Could you check a few things on this model? Use its own coordinates, in mm. Give positions to 0.01 mm unless a question says otherwise; leave off trailing zeros. Order: outer loops, then holes, each group sorted by start corner. A loop starts at its lowest first (then second) coordinate and runs counter-clockwise, first axis right, second up. Notation, with made-up numbers: (9.5, 41) -> (44.5, 41) arc R11 ccw to (44.5, 52) -> close; hole circle Ø1 at (-3, 64.25). An arc over 180 degrees is marked (long way). Use one line per item in the form item = value. Start each with the question number.
from build123d import *

# Parameters (mm, degrees)
SKETCH1_R                  = 19.05
BOSS_EXTRUDE1_DEPTH        = 7.62
SKETCH2_R                  = 2.54
CUT_EXTRUDE1_DEPTH         = 8.62
F_10_24_TAPPED_HOLE1_D     = 3.7973
CIRPATTERN1_COUNT          = 4
F_10_24_TAPPED_HOLE4_D     = 3.7973
F_10_24_TAPPED_HOLE4_DEPTH = 20.0279
F_10_24_TAPPED_HOLE4_TIP   = 1.140824014


with BuildPart() as part:
    # Sketch1 → Boss-Extrude1 (new body)
    with BuildSketch(Plane.XY):
        Circle(SKETCH1_R)
    extrude(amount=BOSS_EXTRUDE1_DEPTH)

    # Sketch2 → Cut-Extrude1 (cut, through all)
    with BuildSketch(Plane.XY.offset(7.62)):
        Circle(SKETCH2_R)
    extrude(amount=-CUT_EXTRUDE1_DEPTH, mode=Mode.SUBTRACT)

    # #10-24 Tapped Hole1 (through all)
    with Locations(Plane.XY.offset(7.62)):
        with Locations((0, 12.7)):
            f_10_24_tapped_hole1 = Hole(F_10_24_TAPPED_HOLE1_D / 2)

    # CirPattern1: #10-24 Tapped Hole1 ×4 about axis
    cirpattern1_axis = Axis((0, 0, 0), (0, 0, 1))
    for i in range(1, CIRPATTERN1_COUNT):
        add(f_10_24_tapped_hole1.rotate(cirpattern1_axis, i * 360 / CIRPATTERN1_COUNT), mode=Mode.SUBTRACT)

    # #10-24 Tapped Hole4
    with Locations(Plane(origin=(13.470384182, 13.470384182, 7.62), x_dir=(-0.707106781, 0.707106781, 0), z_dir=(0.707106781, 0.707106781, 0))):
        with Locations((0, -3.81)):
            Hole(F_10_24_TAPPED_HOLE4_D / 2, depth=F_10_24_TAPPED_HOLE4_DEPTH)
            with Locations((0, 0, -(F_10_24_TAPPED_HOLE4_DEPTH + F_10_24_TAPPED_HOLE4_TIP / 2))):  # 118° drill point
                Cone(0, F_10_24_TAPPED_HOLE4_D / 2, F_10_24_TAPPED_HOLE4_TIP, mode=Mode.SUBTRACT)


solid = part.part
(1) We'd pull the mould along Y, two halves only. Please class faces 1 (the flat face through (4, 0, 7.62)), 2 (the cylindrical face through (-15.12, -11.59, 3.76)), 3 (the cylindrical face through (-0.247, -14.582, 3.757)): pulls with the +Y half, pulls with the -Y half, needs draft (parallel to the pull), parting line crosses it, or undercut.
(2) Please list where these lines run through material, in increasing order: probe 1 along Y at (x, z) = (0, 1.5); probe 2 along Y at (x, z) = (-1.5, 5.5); probe 3 along Y at (x, z) = (11.5, 3.75).
(3) Imagine slicing it at B-B (x = -12.7). Write out the boundary of the cut face in (y, z), plus the area to 3 significant figures.
(4) I'm going to push flat-ended pins straight in: pin 1 Ø3 at (x, y) = (0, -12.7) entering from -Z; pin 2 Ø4 at (y, z) = (-14, 5.5) entering from -X; pin 3 Ø4 at (x, z) = (-10, 5) entering from +Y; pin 4 Ø1 at (y, z) = (9, 5) entering from +X. Where does each tip first touch, or does it pass through?
(5) Imagine slicing it at D-D (x = 1). Give the number of separate pieces and of enclosed holes in the cut face, plus the area to 3 significant figures.
(6) Imagine slicing it at A-A (z = 1.25). Write out the boundary of the cut face in (x, y).
Calculated:
q1.face_1 = needs draft
q1.face_2 = parting line crosses it
q1.face_3 = undercut
q2.probe_1 = -19.05 to -14.6, -10.8 to -2.54, 2.54 to 10.8, 14.6 to 19.05
q2.probe_2 = -18.99 to -13.86, -11.54 to -2.05, 2.05 to 11.54, 13.86 to 18.99
q2.probe_3 = -15.19 to -1.47, 1.47 to 8.82, 14.18 to 15.19
q3.outline = (-14.2, 0) -> (-1.9, 0) -> (-1.9, 7.62) -> (-14.2, 7.62) -> close; (1.9, 0) -> (14.2, 0) -> (14.2, 7.62) -> (1.9, 7.62) -> close
q3.area = 187 mm2
q4.pin_1 = through
q4.pin_2 = -14.8
q4.pin_3 = 17.29
q4.pin_4 = 17.05
q5.separate_pieces = 4
q5.enclosed_holes = 0
q5.area = 202 mm2
q6.outline = circle Ø38.1 at (0, 0); hole circle Ø3.8 at (-12.7, 0); hole circle Ø5.08 at (0, 0); hole circle Ø3.8 at (0, -12.7); hole circle Ø3.8 at (0, 12.7); hole circle Ø3.8 at (12.7, 0)
